Geometry: see drawing. Coordinates: mm, zero at the bounding-box minimum. Give positions to 0.01 mm unless a question says otherwise; leave off trailing zeros. Write each loop counter-clockwise with the first axis right and the second up, starting at its lowest first coordinate (ties: lowest second). Pieces come first, ordered by that corner, then holes. Notation, with made-up numbers: (75, -13) -> (100, -13) arc R29 ccw to (100, 18) -> close; hole circle Ø5 at (74.5, 46.5). An arc over 180 degrees is marked (long way). Write item = value, one per line.
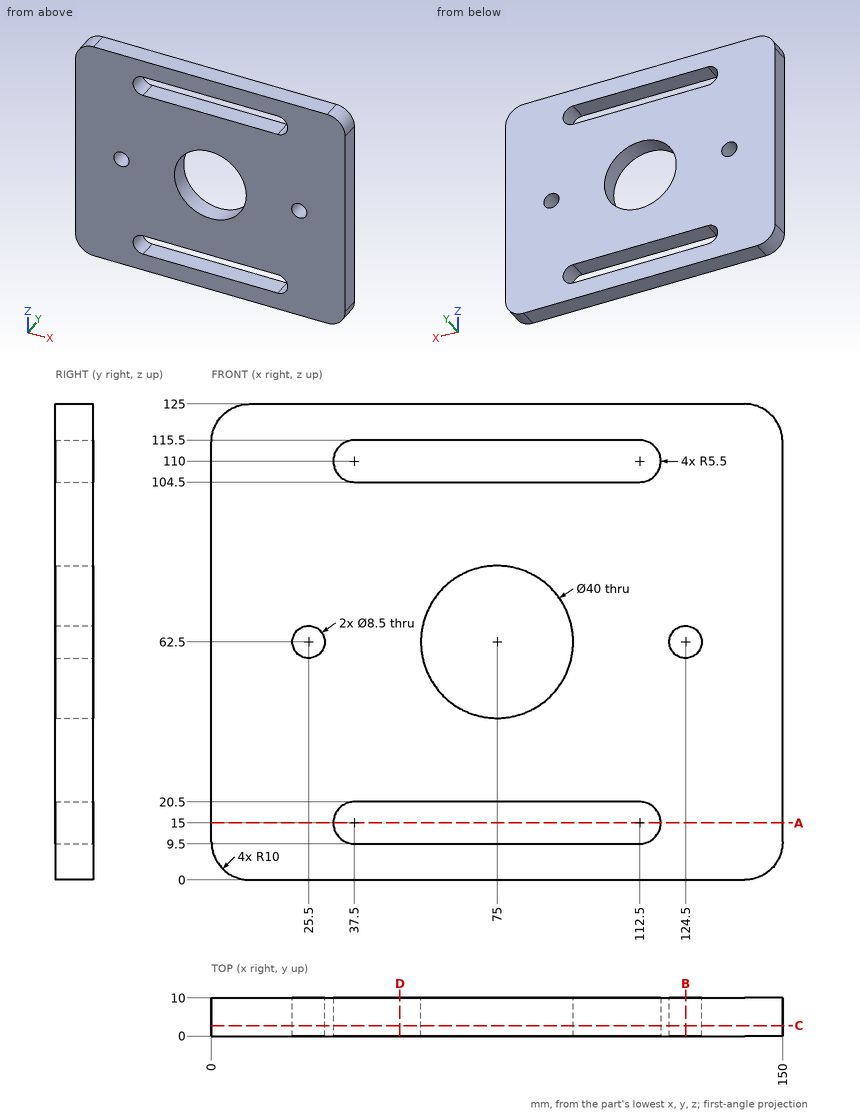
(1) Section query A-A (z = 15). Return loops of the section in (x, y), plus the area to 3 significant figures.
Values follow:
outline = (0, 0) -> (32, 0) -> (32, 10) -> (0, 10) -> close; (118, 0) -> (150, 0) -> (150, 10) -> (118, 10) -> close
area = 640 mm2
(2) Section query C-C (y = 2.75). Return loops of the section in (x, z), plus the area to 3 significant figures.
Values follow:
outline = (0, 10) arc R10 ccw to (10, 0) -> (140, 0) arc R10 ccw to (150, 10) -> (150, 115) arc R10 ccw to (140, 125) -> (10, 125) arc R10 ccw to (0, 115) -> close; hole circle Ø8.5 at (25.5, 62.5); hole (37.5, 9.5) -> (112.5, 9.5) arc R5.5 ccw to (112.5, 20.5) -> (37.5, 20.5) arc R5.5 ccw to start; hole (37.5, 104.5) -> (112.5, 104.5) arc R5.5 ccw to (112.5, 115.5) -> (37.5, 115.5) arc R5.5 ccw to start; hole circle Ø40 at (75, 62.5); hole circle Ø8.5 at (124.5, 62.5)
area = 15,500 mm2
(3) Section query D-D (x = 49.5). Return loops of the section in (y, z).
Values follow:
outline = (0, 0) -> (10, 0) -> (10, 9.5) -> (0, 9.5) -> close; (0, 20.5) -> (10, 20.5) -> (10, 104.5) -> (0, 104.5) -> close; (0, 115.5) -> (10, 115.5) -> (10, 125) -> (0, 125) -> close
(4) Material intervals for line 1 (Z direction, x = 54.5, y = 5.75); line 2 (Z direction, x = 75, y = 5); line 3 (X direction, y = 2, z = 62), sorted ascending.
Values follow:
line_1 = 0 to 9.5, 20.5 to 104.5, 115.5 to 125
line_2 = 0 to 9.5, 20.5 to 42.5, 82.5 to 104.5, 115.5 to 125
line_3 = 0 to 21.28, 29.72 to 55.01, 94.99 to 120.28, 128.72 to 150
(5) Section query B-B (x = 124.5). Return loops of the section in (y, z).
Values follow:
outline = (0, 0) -> (10, 0) -> (10, 58.25) -> (0, 58.25) -> close; (0, 66.75) -> (10, 66.75) -> (10, 125) -> (0, 125) -> close
